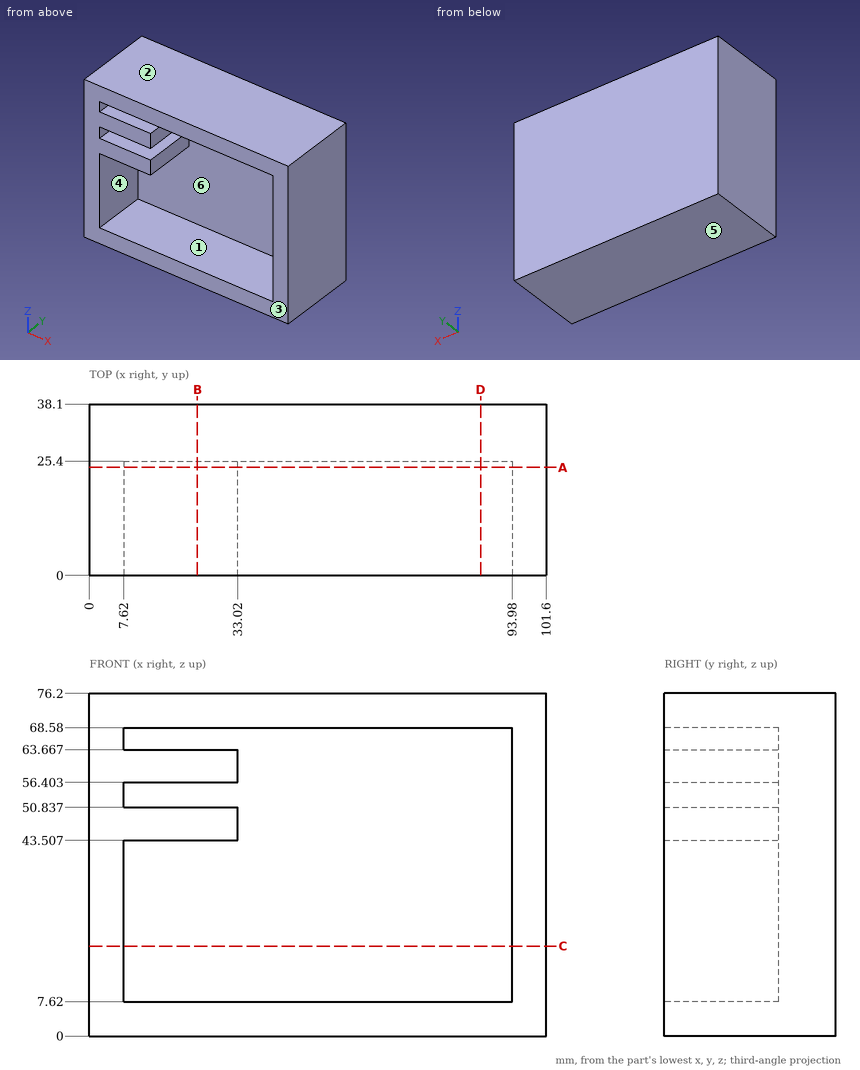
Could you check a few things on this drawing? It's one solid part, dimensions in mm from its lowest x, y, z. A direction names the side the tool comes from. Round coordinates to 2 decimals unless told otherwise and drop trailing zeros. Order: outer loops, then holes, each group sorted by start corner. A loop starts at its lowest first (then second) coordinate and runs counter-clockwise, first axis right, second up. Notation, with made-up numbers: M 1,21.25 L 12,21.25 A20 cw 12,29.25 Z; hole C 4,24 d11. An arc over 180 degrees is marked long. Use a Markdown table: item, result.
1) If I drill on line 1 along Z through (x, y) = (17, 25); line 2 along X through (y, z) = (12.5, 67); line 3 along Z through (x, y) = (36.5, 24), over which ranges is the centre line in solid material (lowest first)?
Geometry says:
| item | result |
|---|---|
| line 1 | z = 0 to 7.62, 43.51 to 50.84, 56.4 to 63.67, 68.58 to 76.2 |
| line 2 | x = 0 to 7.62, 93.98 to 101.6 |
| line 3 | z = 0 to 7.62, 68.58 to 76.2 |
2) Imagine slicing it at C-C (z = 20). List the corners of the cut face in (x, y) for me, then the cut area to 3 significant figures.
Geometry says:
| item | result |
|---|---|
| outline | M 0,0 L 7.62,0 L 7.62,25.4 L 93.98,25.4 L 93.98,0 L 101.6,0 L 101.6,38.1 L 0,38.1 Z |
| area | 1,680 mm² |
3) On a 3-axis mill with a long thin cutter (end or side, diameter ignored), from which of +Z, -Z, +X, -X, +Y, -Y can I reach the whole of each face in a straight line? I mean the marked faces 1 and 2. Say none if no direction works.
Geometry says:
| item | result |
|---|---|
| face 1 | -Y |
| face 2 | +Z, +X, -X, +Y, -Y |
4) I'm going to push a flat-ended pin straight in: P1, Ø6, axis at x = 66.5, z = 54, coming from the -Y side. Where does the tip first touch, or does it pass through?
Geometry says:
| item | result |
|---|---|
| P1 | stops at y = 25.4 |
5) Imagine slicing it at B-B (x = 24). List the corners of the cut face in (y, z) for me, then the cut area to 3 significant figures.
Geometry says:
| item | result |
|---|---|
| outline | M 0,0 L 38.1,0 L 38.1,76.2 L 0,76.2 L 0,68.58 L 25.4,68.58 L 25.4,63.67 L 0,63.67 L 0,56.4 L 25.4,56.4 L 25.4,50.84 L 0,50.84 L 0,43.51 L 25.4,43.51 L 25.4,7.62 L 0,7.62 Z |
| area | 1,730 mm² |
6) Imagine slicing it at D-D (x = 87). List the corners of the cut face in (y, z) for me, then the cut area to 4 significant figures.
Geometry says:
| item | result |
|---|---|
| outline | M 0,0 L 38.1,0 L 38.1,76.2 L 0,76.2 L 0,68.58 L 25.4,68.58 L 25.4,7.62 L 0,7.62 Z |
| area | 1,355 mm² |
7) If we mould it in two halves opening along Z, with no side actions, what happens to the marked faces 3, 4, 5 and 6? For each: +Z half, -Z half, draft (parallel to the pull), parting line (faces both ways), or undercut.
Geometry says:
| item | result |
|---|---|
| face 3 | draft |
| face 4 | undercut |
| face 5 | -Z half |
| face 6 | undercut |
8) Imagine slicing it at A-A (y = 24). List the corners of the cut face in (x, z) for me.
Geometry says:
| item | result |
|---|---|
| outline | M 0,0 L 101.6,0 L 101.6,76.2 L 0,76.2 Z; hole M 7.62,7.62 L 93.98,7.62 L 93.98,68.58 L 7.62,68.58 L 7.62,63.67 L 33.02,63.67 L 33.02,56.4 L 7.62,56.4 L 7.62,50.84 L 33.02,50.84 L 33.02,43.51 L 7.62,43.51 Z |
